```python
from build123d import *

# Parameters (mm, degrees)
HOLE_WIZARD_1_D           = 3.5
HOLE_WIZARD_1_CBORE_D     = 6
HOLE_WIZARD_1_CBORE_DEPTH = 4
PATTERN_CIRCULAR_1_COUNT  = 6
CHAMFER_1_SIZE            = 0.5


with BuildPart() as part:
    # 草图1 → 旋转1 (revolve)
    with BuildSketch(Plane(origin=(0, 0, 0), x_dir=(0, 0, -1), z_dir=(1, 0, 0))):
        Polygon((-15, 75), (-15, 0), (-30, 0), (-30, 7.5), (-22.5, 7.5), (-22.5, 35), (-20, 35), (-20, 60), (-17.5, 60), (-17.5, 75), align=None)
    revolve(axis=Axis((0, 44, 0), (0, -1, 0)))

    # 打孔尺寸(%根据)内六角圆柱头螺钉的类型1 (through all)
    with Locations(Plane(origin=(0, 0, 0), x_dir=(-1, 0, 0), z_dir=(0, -1, 0))):
        with Locations((0, -25)):
            hole_wizard_1 = CounterBoreHole(HOLE_WIZARD_1_D / 2, HOLE_WIZARD_1_CBORE_D / 2, HOLE_WIZARD_1_CBORE_DEPTH)

    # 阵列(圆周)1: 打孔尺寸(%根据)内六角圆柱头螺钉的类型1 ×6 about axis
    pattern_circular_1_axis = Axis((0, 0, 0), (0, 1, 0))
    for i in range(1, PATTERN_CIRCULAR_1_COUNT):
        add(hole_wizard_1.rotate(pattern_circular_1_axis, i * 360 / PATTERN_CIRCULAR_1_COUNT), mode=Mode.SUBTRACT)

    # 倒角1
    chamfer_1_edges = [part.edges().sort_by_distance(p)[0] for p in [
        (0, 7.5, -30),
        (0, 0, -30),
        (0, 75, -17.5),
    ]]
    chamfer(chamfer_1_edges, length=CHAMFER_1_SIZE)


solid = part.part
```
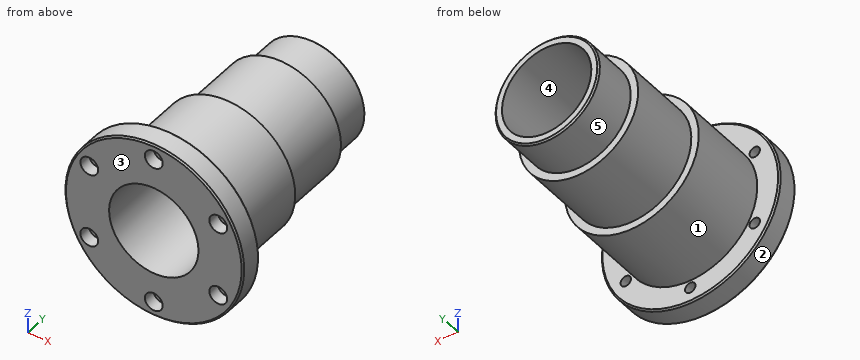
Geometry check sheet. Reference: the model listing, model coordinates, mm. Face numbers are marked on the shaded views. A direction names the side the tool comes from. Coordinates: 2 decimals unless noted, no trailing zeros. Loops run counter-clockwise (first coordinate to the right, second up) from the corner with the lowest first, then second, coordinate; pieces in that order, holes last. Notation, with made-up numbers: (-18.75, -19.75) - (-12.75, -19.75) arc R12 cw to (-12.75, -0.75) - close; hole circle Ø7 at (69, 85). An arc over 180 degrees is marked (long way). One line per item, written item: value. Start each with the question number.
(1) Depth check by flat-ended pin: P1, Ø1.8, axis at x = -23, z = 12, coming from the -Y side; P2, Ø1.8, axis at x = 22, z = -12, coming from the -Y side; P3, Ø5.5, axis at x = -21.65, z = 12.5, coming from the +Y side; P4, Ø3, axis at y = 24, z = -19, coming from the +X side. Enter the tip coordinate at first touch or a pass-through.
(2) Cross-section at B-B on x = 0. Count the separate pieces of the cut face and the enclosed holes in it, plus the area to 3 significant figures.
(3) Tool access check on the marked faces 1 and 2. Record the directions out of +Z, -Z, +X, -X, +Y, -Y that give a thin tool (end or side, any length) a straight path to the whole face; none if there is none.
(4) Cross-section at C-C on y = 15. Enter the section's corners in (x, z).
(5) Cross-section at A-A on z = 0. Enter the section's corners in (x, y), plus the area to 3 significant figures.
(6) Mould release check, pull along Z, two halves, no side actions. Record for the marked faces 3, 4 and 5: released by +Z, released by -Z, zero draft, split by the parting line, or undercut.
(7) Material ranges on line 1 (X direction, y = 44.5, z = 0); line 2 (Y direction, x = 11, z = -15.5); line 3 (Y direction, x = 16.5, z = 21), recorded low to high. Write a range as [from, to].
Results below:
1. P1: stops at y = 4
1. P2: passes through
1. P3: stops at y = 35
1. P4: stops at x = 14.14
2. separate pieces: 4
2. enclosed holes: 0
2. area: 889 mm2
3. face 1: +Y
3. face 2: +Y, -Y
4. outline: circle Ø45 at (0, 0); hole circle Ø30 at (0, 0)
5. outline: (-30, 0.5) - (-29.5, 0) - (-15, 0) - (-15, 75) - (-17, 75) - (-17.5, 74.5) - (-17.5, 60) - (-20, 60) - (-20, 35) - (-22.5, 35) - (-22.5, 7.5) - (-29.5, 7.5) - (-30, 7) - close; (15, 0) - (29.5, 0) - (30, 0.5) - (30, 7) - (29.5, 7.5) - (22.5, 7.5) - (22.5, 35) - (20, 35) - (20, 60) - (17.5, 60) - (17.5, 74.5) - (17, 75) - (15, 75) - close
5. area: 962 mm2
6. face 3: zero draft
6. face 4: undercut
6. face 5: split by the parting line
7. line 1: x = [-20, -15], [15, 20]
7. line 2: y = [0, 60]
7. line 3: y = [0, 7.5]
